```python
from build123d import *

# Parameters (mm, degrees)
SKETCH1_R           = 5.5
SKETCH1_R_2         = 1.1
BOSS_EXTRUDE1_DEPTH = 2
BOSS_EXTRUDE3_START = -2
BOSS_EXTRUDE3_DEPTH = 2


with BuildPart() as part:
    # Sketch1 → Boss-Extrude1 (new body)
    with BuildSketch(Plane.XY):
        Circle(SKETCH1_R)
        Circle(SKETCH1_R_2, mode=Mode.SUBTRACT)
    extrude(amount=BOSS_EXTRUDE1_DEPTH)

    # Sketch2 → Boss-Extrude3 (add)
    with BuildSketch(Plane.XY.offset(2).offset(BOSS_EXTRUDE3_START)):
        with BuildLine():
            Line((-0.9, 0.632455532), (0.9, 0.632455532))
            ThreePointArc((0.9, 0.632455532), (0, 1.1), (-0.9, 0.632455532))
        make_face()
    extrude(amount=BOSS_EXTRUDE3_DEPTH)

    # Sketch3 → Cut-Revolve1 (revolve, cut)
    with BuildSketch(Plane(origin=(0, 0, 0), x_dir=(0, 0, -1), z_dir=(1, 0, 0)), mode=Mode.PRIVATE) as cut_revolve1_sk:
        with BuildLine():
            Line((-0.05, 5.5), (-1.95, 5.5))
            ThreePointArc((-1.95, 5.5), (-1, 4.55), (-0.05, 5.5))
        make_face()
    revolve(cut_revolve1_sk.sketch.rotate(Axis((0, 0, -0.1), (0, 0, 1)), 90), axis=Axis((0, 0, -0.1), (0, 0, 1)), mode=Mode.SUBTRACT)


solid = part.part
```
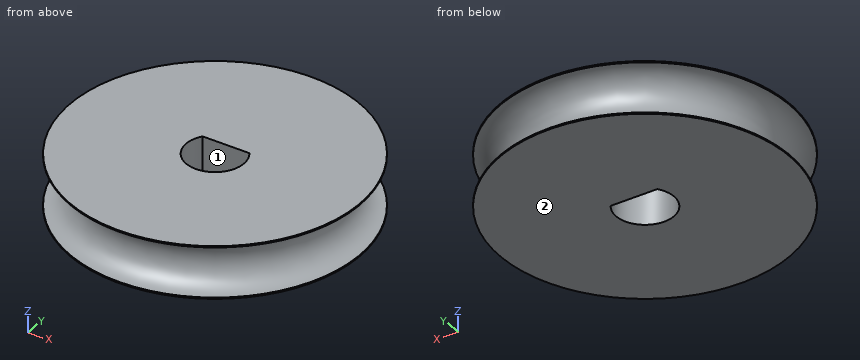
Model file for the job. Use its own axes, mm. Face numbers are marked on the shaded views. Coordinates: 2 decimals unless noted, no trailing zeros. Order: outer loops, then holes, each group sorted by start corner. A loop starts at its lowest first (then second) coordinate and runs counter-clockwise, first axis right, second up. Notation, with made-up numbers: (-23.75, -38.5) -> (5.25, -38.5) arc R18 ccw to (5.25, -3.5) -> close; hole circle Ø10 at (81.25, -38.5). An arc over 180 degrees is marked (long way). Answer as a JSON object with one key per item and string values. Group by question number.
1) Cut at A-A, the plane y = 0. Write the cut outline in (x, z), then the cut area to 3 significant figures.
2) Cut at B-B, the plane x = 0. Write the cut outline in (y, z).
3) Drill centre lines: L1, parallel to X at y = -0.25, z = 0.7; L2, parallel to Z at x = -3.75, y = 3; L3, parallel to X at y = -0.25, z = 0.3. Where is each one in solid material? Low to high.
4) Cut at C-C, the plane z = 0.25. Write the cut outline in (x, y).
5) Flat gauge pin, fed straight in: pin 1 (1 mm diameter, centred on x = -1.5, z = 1.5, fed in from +Y). Where does the tip first touch, or does it go through?
6) Pull direction X, two halves, no side cores. Call the marked faces 1 and 2: +X half, -X half, draft (parallel to the pull), parting line (faces both ways), or undercut.
Check values:
{
 "1": {"outline": "(-5.5, 0) -> (-1.1, 0) -> (-1.1, 2) -> (-5.5, 2) -> (-5.5, 1.95) arc R0.95 cw to (-5.5, 0.05) -> close; (1.1, 0) -> (5.5, 0) -> (5.5, 0.05) arc R0.95 cw to (5.5, 1.95) -> (5.5, 2) -> (1.1, 2) -> close", "area": "14.8 mm²"},
 "2": {"outline": "(-5.5, 0) -> (-1.1, 0) -> (-1.1, 2) -> (-5.5, 2) -> (-5.5, 1.95) arc R0.95 cw to (-5.5, 0.05) -> close; (0.63, 0) -> (5.5, 0) -> (5.5, 0.05) arc R0.95 cw to (5.5, 1.95) -> (5.5, 2) -> (0.63, 2) -> close"},
 "3": {"L1": "x = -4.59 to -1.07, 1.07 to 4.59", "L2": "z = 0 to 0.36, 1.64 to 2", "L3": "x = -4.85 to -1.07, 1.07 to 4.85"},
 "4": {"outline": "circle Ø9.83 at (0, 0); hole (-0.9, 0.63) arc R1.1 ccw (long way) to (0.9, 0.63) -> close"},
 "5": {"pin 1": "stops at y = 5.35"},
 "6": {"face 1": "undercut", "face 2": "draft"}
}
